```python
from build123d import *

# Parameters (mm, degrees)
F0_R     = 1.9
F1_DEPTH = 5
F0_W     = 10
F0_H     = 40
F2_DEPTH = 25
F3_R     = 2.8
F4_DEPTH = 10


with BuildPart() as f1:
    # F0 (on Top) → F1 (new body)
    with BuildSketch(Plane.XY):
        Polygon((20.990842, 38.977277), (-37.259158, 38.977277), (-37.259158, 7.727277), (-27.259158, 7.727277), (-27.259158, 28.977277), (10.990842, 28.977277), (10.990842, -53.522723), (-27.259158, -53.522723), (-27.259158, -32.272723), (-37.259158, -32.272723), (-37.259158, -63.522723), (20.990842, -63.522723), align=None)
        with Locations((-32.259158, -46.022723)):
            Circle(F0_R, mode=Mode.SUBTRACT)
        with Locations((15.990842, -53.522723)):
            Circle(F0_R, mode=Mode.SUBTRACT)
        with Locations((-32.259158, 28.977277)):
            Circle(F0_R, mode=Mode.SUBTRACT)
        with Locations((15.990842, 28.977277)):
            Circle(F0_R, mode=Mode.SUBTRACT)
    extrude(amount=F1_DEPTH)

    # F0 (on Top) → F2 (join)
    with BuildSketch(Plane.XY):
        with Locations((-32.259158, -12.272723)):
            Rectangle(F0_W, F0_H)
    extrude(amount=F2_DEPTH)

    # F3 (on face) → F4 (cut, through all)
    with BuildSketch(Plane(origin=(-37.259158, 0, 0), x_dir=(0, -1, 0), z_dir=(-1, 0, 0))):
        with Locations((2.272723, 15)):
            Circle(F3_R)
        with Locations((22.272723, 15)):
            Circle(F3_R)
    extrude(amount=-F4_DEPTH, mode=Mode.SUBTRACT)


solid = f1.part
```
Model file for the job. Use its own axes, mm. A direction names the side the tool comes from. Give positions to 0.01 mm unless a question says otherwise; leave off trailing zeros. Write each loop counter-clockwise with the first axis right and the second up, starting at its lowest first coordinate (ties: lowest second). Pieces come first, ordered by that corner, then holes. Notation, with made-up numbers: (-3.75, 30.25) -> (12.25, 30.25) arc R14 ccw to (12.25, 46.25) -> close; hole circle Ø1 at (88, 77). An arc over 180 degrees is marked (long way). Use CSV: the item, a comma, the result in double quotes. Start each with the question number.
1) Cut at B-B on y = 10.5. List the corners of the cut face in (x, z), plus the area to 3 significant figures.
2) Two-plate mould, pull along Y, no slides. Class faces 4 (the cylindrical face through (-34.157, -45.939, 2.465)), 5 (the flat face through (-8, 38.977, 2)), 6 (the flat face through (-28, -12, 0)): released by +Y, released by -Y, zero draft, split by the parting line, or undercut.
3) Pin check, flat tips, straight feed: P1, Ø3.5, axis at x = -32.26, y = 28.98, coming from the +Z side; P2, Ø8, axis at x = -31.5, z = 17, coming from the +Y side; P3, Ø6.5, axis at y = -2.27, z = 15, coming from the +X side; P4, Ø4.5, axis at x = 15.99, y = 28.98, coming from the -Z side. Stop position of each tip, or through.
4) Drill centre lines: L1, parallel to Y at x = -8, z = 1.25; L2, parallel to X at y = 6, z = 6.25; L3, parallel to X at y = 27, z = 2. Where is each one in solid material? Low to high.
5) Tool access for faces 1 (the cylindrical face through (-32.329, -1.666, 12.267)), 2 (the flat face through (-32, 7.727, 15)), 3 (the flat face through (-8, 28.977, 2)): list every direction of +Z, -Z, +X, -X, +Y, -Y with a clear straight run to the whole face (end or side of a thin tool).
6) Cut at D-D on y = -2.5. List the corners of the cut face in (x, z), plus the area to 3 significant figures.
7) Cut at A-A on x = -8.5. List the corners of the cut face in (y, z), plus the area to 3 significant figures.
8) Cut at C-C on z = 15. List the corners of the cut face in (x, y), plus the area to 3 significant figures.
Final values:
1,outline,"(-37.26, 0) -> (-27.26, 0) -> (-27.26, 5) -> (-37.26, 5) -> close; (10.99, 0) -> (20.99, 0) -> (20.99, 5) -> (10.99, 5) -> close"
1,area,"100 mm2"
2,face 4,"undercut"
2,face 5,"released by +Y"
2,face 6,"zero draft"
3,P1,"passes through"
3,P2,"stops at y = 7.73"
3,P3,"stops at x = -27.26"
3,P4,"stops at z = 0"
4,L1,"y = -63.52 to -53.52, 28.98 to 38.98"
4,L2,"x = -37.26 to -27.26"
4,L3,"x = -37.26 to -27.26, 10.99 to 20.99"
5,face 1,"+X, -X"
5,face 2,"+Z, +X, -X, +Y"
5,face 3,"+Z, -Z"
6,outline,"(-37.26, 0) -> (-27.26, 0) -> (-27.26, 12.21) -> (-37.26, 12.21) -> close; (-37.26, 17.79) -> (-27.26, 17.79) -> (-27.26, 25) -> (-37.26, 25) -> close; (10.99, 0) -> (20.99, 0) -> (20.99, 5) -> (10.99, 5) -> close"
6,area,"244 mm2"
7,outline,"(-63.52, 0) -> (-53.52, 0) -> (-53.52, 5) -> (-63.52, 5) -> close; (28.98, 0) -> (38.98, 0) -> (38.98, 5) -> (28.98, 5) -> close"
7,area,"100 mm2"
8,outline,"(-37.26, -32.27) -> (-27.26, -32.27) -> (-27.26, -25.07) -> (-37.26, -25.07) -> close; (-37.26, -19.47) -> (-27.26, -19.47) -> (-27.26, -5.07) -> (-37.26, -5.07) -> close; (-37.26, 0.53) -> (-27.26, 0.53) -> (-27.26, 7.73) -> (-37.26, 7.73) -> close"
8,area,"288 mm2"
